The figure shows three views and two pictorial views of one solid part (mm, origin at its lowest corner). Answer the questions. Coordinates: 2 decimals unless noted, no trailing zeros. Order: outer loops, then holes, each group sorted by start corner. A loop starts at its lowest first (then second) coordinate and runs counter-clockwise, first axis right, second up. Notation, with made-up numbers: M 60,6 L 112,6 A28 ccw 112,27 Z; hole C 18,54 d10. An arc over 180 degrees is marked long. Write item = value, one per line. Start each with the question number.
Q1. Find section B-B on z = 49.5. Give the vertices of the cut face in (x, y), and give its area (3 significant figures).
Q2. Find section C-C on x = 16. Give the vertices of the cut face in (y, z).
Q3. Find section D-D on y = 0.6. Give the number of separate pieces and of enclosed holes in the cut face, and give its area (3 significant figures).
Q4. Find section A-A on x = 31. Give the vertices of the cut face in (y, z), and give its area (3 significant figures).
Q5. Straight lines are drawn through the part: line 1 along X through (y, z) = (0.55, 7.5); line 2 along Z through (x, y) = (13, 0.5); line 3 along Z through (x, y) = (17, 0.8). For each, find the intervals that lie inside material, in ascending order.
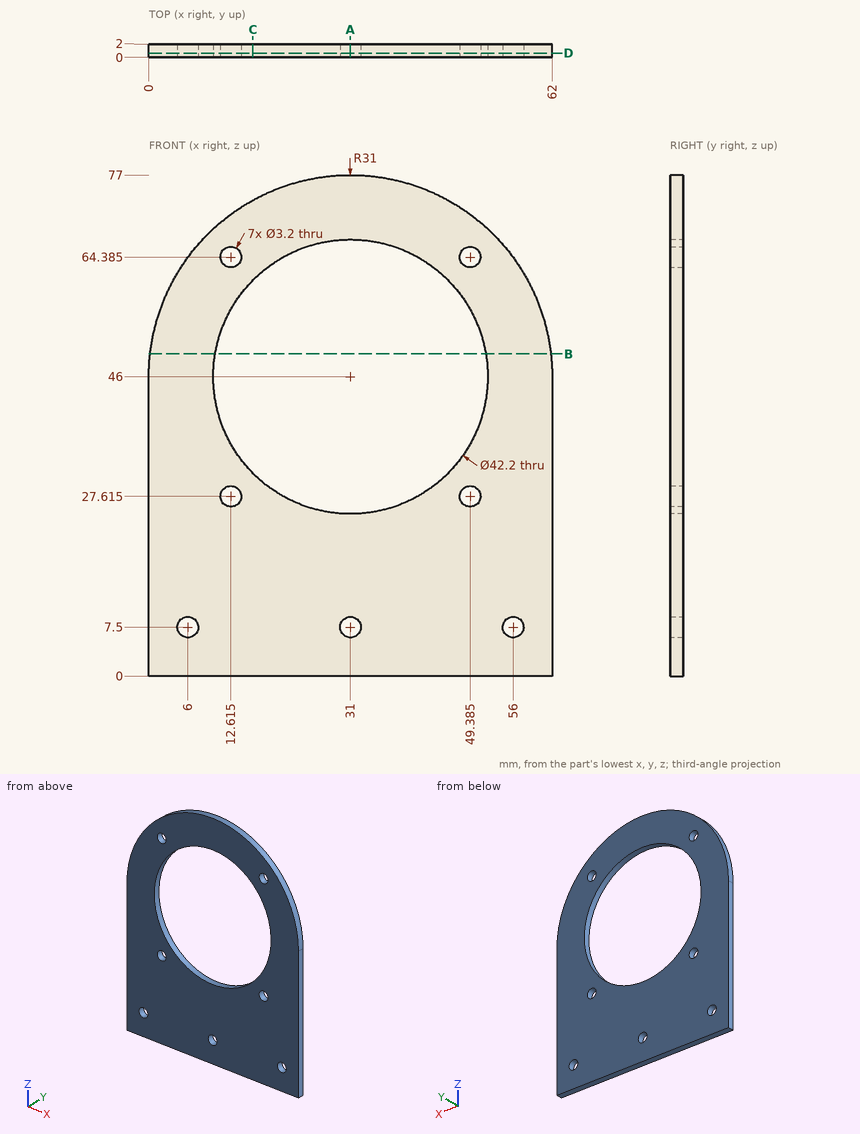
Findings below:
q1.outline = M 0.2,0 L 10.19,0 L 10.19,2 L 0.2,2 Z; M 51.81,0 L 61.8,0 L 61.8,2 L 51.81,2 Z
q1.area = 40.0 mm^2
q2.outline = M 0,0 L 2,0 L 2,31.16 L 0,31.16 Z; M 0,60.84 L 2,60.84 L 2,73.13 L 0,73.13 Z
q3.separate_pieces = 1
q3.enclosed_holes = 8
q3.area = 2,910 mm^2
q4.outline = M 0,0 L 2,0 L 2,5.9 L 0,5.9 Z; M 0,9.1 L 2,9.1 L 2,24.9 L 0,24.9 Z; M 0,67.1 L 2,67.1 L 2,77 L 0,77 Z
q4.area = 63.2 mm^2
q5.line_1 = 0 to 4.4, 7.6 to 29.4, 32.6 to 54.4, 57.6 to 62
q5.line_2 = 0 to 26.06, 29.17 to 34.99, 57.01 to 62.83, 65.94 to 71.24
q5.line_3 = 0 to 30.21, 61.79 to 73.66
